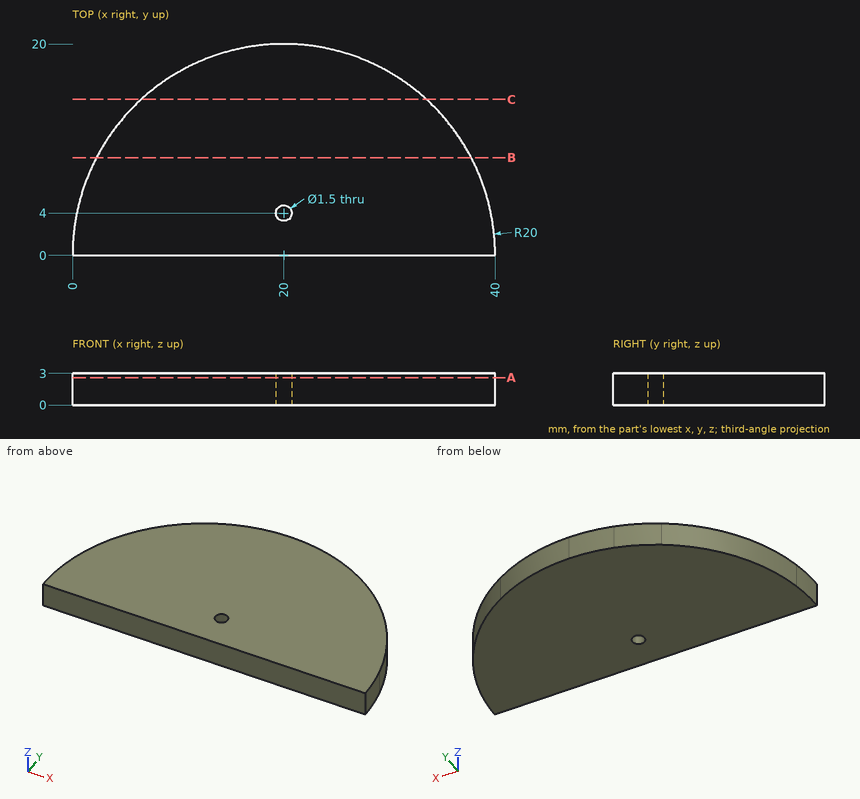
Input: dimensioned drawing with shaded views. Units: mm. Origin: part minimum x, y, z. Give positions to 0.01 mm unless a question says otherwise; leave off trailing zeros. Write each loop counter-clockwise with the first axis right and the second up, starting at its lowest first coordinate (ties: lowest second). Pieces come first, ordered by that corner, then holes. Notation, with made-up numbers: (74.5, -23.75) - (116.5, -23.75) arc R22 ccw to (116.5, -8.75) - close; hole circle Ø1 at (66, 49). An arc over 180 degrees is marked (long way). One line per item, written item: value. Start each with the question number.
Q1. Material intervals for probe 1 along Y at (x, z) = (20, 0.95); probe 2 along X at (y, z) = (4.5, 1.9); probe 3 along Y at (x, z) = (36, 1.6), sorted ascending. Write a range as from..to.
Q2. First-contact query: pin 1 Ø1.2 at (x, y) = (20, 4) entering from -Z. Flat tip, straight axial feed; report the tip coordinate or a pass-through.
Q3. Section query B-B, the plane y = 9.25. Return the cut outline in (x, z), then the cut area to 3 significant figures.
Q4. Section query A-A, the plane z = 2.6. Return the cut outline in (x, y).
Q5. Section query C-C, the plane y = 14.75. Return the cut outline in (x, z), then the cut area to 3 significant figures.
Answer:
1. probe 1: y = 0..3.25, 4.75..20
1. probe 2: x = 0.51..19.44, 20.56..39.49
1. probe 3: y = 0..12
2. pin 1: passes through
3. outline: (2.27, 0) - (37.73, 0) - (37.73, 3) - (2.27, 3) - close
3. area: 106 mm2
4. outline: (0, 0) - (40, 0) arc R20 ccw to start; hole circle Ø1.5 at (20, 4)
5. outline: (6.49, 0) - (33.51, 0) - (33.51, 3) - (6.49, 3) - close
5. area: 81.0 mm2
